Could you check a few things on this model? Use its own coordinates, in mm. A direction names the side the tool comes from. Give positions to 0.01 mm unless a question says otherwise; leave off trailing zeros. Order: outer loops, then holes, each group sorted by start corner. A loop starts at its lowest first (then second) coordinate and runs counter-clockwise, first axis right, second up. Notation, with made-up numbers: (31, -6.5) -> (36, -6.5) arc R14 ccw to (36, 20.5) -> close; hole circle Ø9 at (67.25, 33.25). An arc over 180 degrees is marked (long way). Use one line per item in the form item = value. Start each with the question number.
from build123d import *

# Parameters (mm, degrees)
BOSS_EXTRUDE1_DEPTH = 3


with BuildPart() as part:
    # Sketch1 → Boss-Extrude1 (new body)
    with BuildSketch(Plane(origin=(0, 0, 0), x_dir=(0, 0, -1), z_dir=(1, 0, 0))):
        Polygon((10, 153.005875518), (20, 153.005875518), (20, 150.005875518), (30, 150.005875518), (30, 153.005875518), (40, 153.005875518), (40, 150.005875518), (50, 150.005875518), (50, 153.005875518), (60, 153.005875518), (60, 150.005875518), (70, 150.005875518), (70, 146.5), (70, 143.5), (70, 140), (73, 140), (73, 130), (70, 130), (70, 120), (73, 120), (73, 110), (70, 110), (70, 100), (73, 100), (73, 90), (70, 90), (70, 83.5), (70, 80), (73, 80), (73, 70), (70, 70), (70, 66.5), (70, 63.5), (70, 60), (73, 60), (73, 50), (70, 50), (70, 40), (73, 40), (73, 30), (70, 30), (70, 20), (73, 20), (73, 10), (70, 10), (70, 6.5), (70, 3.5), (70, 0), (60, 0), (60, -3), (50, -3), (50, 0), (40, 0), (40, -3), (30, -3), (30, 0), (20, 0), (20, -3), (10, -3), (10, 0), (0, 0), (0, 3.5), (5, 3.5), (5, 2.5), (7.5, 2.5), (7.5, 3.5), (16, 3.5), (16, 6.5), (7.5, 6.5), (7.5, 7.5), (5, 7.5), (5, 6.5), (0, 6.5), (0, 10), (-3, 10), (-3, 20), (0, 20), (0, 30), (-3, 30), (-3, 40), (0, 40), (0, 50), (-3, 50), (-3, 60), (0, 60), (0, 63.5), (5, 63.5), (5, 62.5), (7.5, 62.5), (7.5, 63.5), (16, 63.5), (16, 66.5), (7.5, 66.5), (7.5, 67.5), (5, 67.5), (5, 66.5), (0, 66.5), (0, 70), (-3, 70), (-3, 80), (0, 80), (0, 83.5), (5, 83.5), (5, 82.5), (7.5, 82.5), (7.5, 83.5), (16, 83.5), (16, 86.5), (7.5, 86.5), (7.5, 87.5), (5, 87.5), (5, 86.5), (0, 86.5), (0, 90), (-3, 90), (-3, 100), (0, 100), (0, 110), (-3, 110), (-3, 120), (0, 120), (0, 130), (-3, 130), (-3, 140), (0, 140), (0, 143.5), (5, 143.5), (5, 142.5), (7.5, 142.5), (7.5, 143.5), (16, 143.5), (16, 146.5), (7.5, 146.5), (7.5, 147.5), (5, 147.5), (5, 146.5), (0, 146.5), (0, 150.005875518), (10, 150.005875518), align=None)
    extrude(amount=BOSS_EXTRUDE1_DEPTH)


solid = part.part
(1) Imagine slicing it at A-A (z = -27.5). Write out the boundary of the cut face in (x, y).
(2) Which directions (+Z, -Z, +X, -X, +Y, -Y) give clear straight access to the entire face, cutting with the end or side of a thin tool? Please do faces 4 (the flat face through (1, 150.006, -45)), 5 (the flat face through (1, -1, -40)), 6 (the flat face through (1, 30, -72)).
(3) I'm going to push flat-ended pins straight in: pin 1 Ø1.5 at (x, z) = (2, -3.5) entering from +Y; pin 2 Ø8 at (y, z) = (108, -23.5) entering from -X; pin 3 Ø1.1 at (x, y) = (2, 143) entering from +Z; pin 4 Ø0.9 at (x, y) = (1, 44) entering from -Z. Where does each tip first touch, or does it pass through?
(4) Please list where these lines run through material, in increasing order: probe 1 along Y at (x, z) = (2.25, -9); probe 2 along Y at (x, z) = (0.8, -15); probe 3 along Y at (x, z) = (1.9, -23).
(5) We'd pull the mould along Y, two halves only. Please class faces 1 (the flat face through (1, 135, 3)), 2 (the flat face through (1, 140, 2)), 3 (the flat face through (1, 40, -71)): pulls with the +Y half, pulls with the -Y half, needs draft (parallel to the pull), parting line crosses it, or undercut.
(6) Imagine slicing it at B-B (y = 27). Write out the boundary of the cut face in (x, z), plus the area to 3 significant figures.
Calculated:
q1.outline = (0, 0) -> (3, 0) -> (3, 150.01) -> (0, 150.01) -> close
q2.face_4 = +X, -X, +Y
q2.face_5 = +X, -X, -Y
q2.face_6 = -Z, +X, -X
q3.pin_1 = 150.01
q3.pin_2 = 0
q3.pin_3 = 0
q3.pin_4 = -70
q4.probe_1 = 0 to 3.5, 6.5 to 63.5, 66.5 to 83.5, 86.5 to 143.5, 146.5 to 150.01
q4.probe_2 = -3 to 3.5, 6.5 to 63.5, 66.5 to 83.5, 86.5 to 143.5, 146.5 to 153.01
q4.probe_3 = 0 to 150.01
q5.face_1 = needs draft
q5.face_2 = pulls with the +Y half
q5.face_3 = undercut
q6.outline = (0, -70) -> (3, -70) -> (3, 0) -> (0, 0) -> close
q6.area = 210 mm2
